from build123d import *

# Parameters (mm, degrees)
CUT_EXTRUDE1_DEPTH = 1.5


with BuildPart() as part:
    # Sketch1 → Revolve1 (revolve)
    with BuildSketch(Plane.XY, mode=Mode.PRIVATE) as revolve1_sk:
        Polygon((-2, 0), (-2, 2.75), (0, 2.75), (0, 1.5), (10, 1.5), (10, 0), align=None)
    revolve(revolve1_sk.sketch.rotate(Axis((-22.358139419, 0, 0), (1, 0, 0)), 90), axis=Axis((-22.358139419, 0, 0), (1, 0, 0)))

    # Sketch2 → Cut-Revolve1 (revolve, cut)
    with BuildSketch(Plane(origin=(0, 0, 0), x_dir=(1, 0, 0), z_dir=(0, 1, 0)), mode=Mode.PRIVATE) as cut_revolve1_sk:
        Polygon((-2, 1.25), (-2, 0), (0.221687836, 0), (-0.5, 1.25), align=None)
    revolve(cut_revolve1_sk.sketch.rotate(Axis((-5.673571921, 0, 0), (1, 0, 0)), 180), axis=Axis((-5.673571921, 0, 0), (1, 0, 0)), mode=Mode.SUBTRACT)

    # Sketch3 → Cut-Extrude1 (cut)
    with BuildSketch(Plane.ZY.offset(2)):
        Polygon((0, 1.443375673), (-1.25, 0.721687836), (-1.25, -0.721687836), (0, -1.443375673), (1.25, -0.721687836), (1.25, 0.721687836), align=None)
    extrude(amount=-CUT_EXTRUDE1_DEPTH, mode=Mode.SUBTRACT)


solid = part.part
Geometry check sheet. Reference: the model listing, model coordinates, mm. A direction names the side the tool comes from. Give positions to 0.01 mm unless a question says otherwise; leave off trailing zeros. Loops run counter-clockwise (first coordinate to the right, second up) from the corner with the lowest first, then second, coordinate; pieces in that order, holes last. Notation, with made-up numbers: M 68,-5.75 L 76,-5.75 A14 cw 76,18.25 Z; hole C 22,50.25 d8. An arc over 180 degrees is marked long. Answer as a JSON object with one key per item and string values. Group by question number.
Item 1: Sectioned sample at A-A on x = -0.25. Record the boundary of the cut face in (y, z).
Item 2: Gauge pin test, flat ends, axial feed: pin 1 (1 mm diameter, centred on x = 1.5, y = 1.5, fed in from -Z); pin 2 (1.5 mm diameter, centred on x = 3.5, y = 2, fed in from +Z). Record the tip position at first contact, or that the pin passes through.
Item 3: Access from +Z, -Z, +X, -X, +Y, -Y to the whole of each face (thin tool, end or side, straight path). Record for faces 1 (the flat face through (-2, -1.3, -0.6)), 2 (the flat face through (-1.26, -1.08, -0.63)), 3 (the flat face through (0, 1.2, 1.2)).
Item 4: Material ranges on L1, parallel to Z at x = 9, y = -0.05; L2, parallel to X at y = 2.05, z = -0.4; L3, parallel to Y at x = 4.25, z = -1.3, recorded low to high.
Item 5: Mould release check, pull along Y, two halves, no side actions. Record for faces 4 (the flat face through (10, 0, 0)), 5 (the flat face through (-1.26, 1.08, 0.63)), 6 (the cylindrical face through (-0.986, 2.685, -0.596)): pulls with the +Y half, pulls with the -Y half, needs draft (parallel to the pull), parting line crosses it, or undercut.
Item 6: Sectioned sample at D-D on z = 1.8. Record the boundary of the cut face in (x, y).
Item 7: Sectioned sample at B-B on x = 6. Record the boundary of the cut face in (y, z).
Item 8: Sectioned sample at C-C on y = 2. Record the boundary of the cut face in (x, z), plus the area to 3 significant figures.
Findings below:
{
 "1": {"outline": "C 0,0 d5.5; hole C 0,0 d1.63"},
 "2": {"pin 1": "z = -1.12", "pin 2": "z = 0.83"},
 "3": {"face 1": "+Z, -Z, -X, +Y, -Y", "face 2": "-X", "face 3": "+X"},
 "4": {"L1": "-1.5 to 1.5", "L2": "-2 to 0", "L3": "-0.75 to 0.75"},
 "5": {"face 4": "needs draft", "face 5": "undercut", "face 6": "parting line crosses it"},
 "6": {"outline": "M -2,-2.08 L 0,-2.08 L 0,2.08 L -2,2.08 Z"},
 "7": {"outline": "C 0,0 d3"},
 "8": {"outline": "M -2,-1.89 L 0,-1.89 L 0,1.89 L -2,1.89 Z", "area": "7.55 mm2"}
}
